For this review, use the dimensioned drawing (mm, ordinates from the lowest corner) and the shaded views. A direction names the side the tool comes from. Give positions to 0.01 mm unless a question says otherwise; leave off trailing zeros. Order: outer loops, then holes, each group sorted by start corner. A loop starts at its lowest first (then second) coordinate and runs counter-clockwise, first axis right, second up. Notation, with made-up numbers: (41, 84) - (87, 84) arc R19 ccw to (87, 99) - close; hole circle Ø10 at (79, 23). An arc over 180 degrees is marked (long way). Use a Markdown table: item, result. Add a question column.
1) We need section D-D on y = 24.5. Write out the cut boundary in (x, z), then the cut area to 3 significant figures.
2) We need section A-A on y = 39.5. Write out the cut boundary in (x, z).
3) Machinability: for the marked faces 1, 2, 3, 4 and 5, which of the approach directions +Z, -Z, +X, -X, +Y, -Y give a long, thin tool a straight path to every point of the face, cutting with its end or side? Answer none if there is none.
4) Clearance check with flat-ended pins moving along their axes: P1, Ø20.5, axis at y = 50, z = 43, coming from the +X side; P2, Ø1, axis at x = 47.5, y = 33.5, coming from the -Z side; P3, Ø15, axis at y = 47.5, z = 35, coming from the -X side. State where each tip first meets the part, or that it passes through.
5) We need section B-B on z = 65.5. Write out the cut boundary in (x, y), then the cut area to 3 significant figures.
6) We need section C-C on x = 20. Write out the cut boundary in (y, z), then the cut area to 3 significant figures.
7) Wall thickness on L1, parallel to Y at x = 94, z = 67.5; L2, parallel to Z at x = 58, y = 24; L3, parallel to Z at x = 133, y = 18: over which ranges is each line inside the solid? List them lowest first.
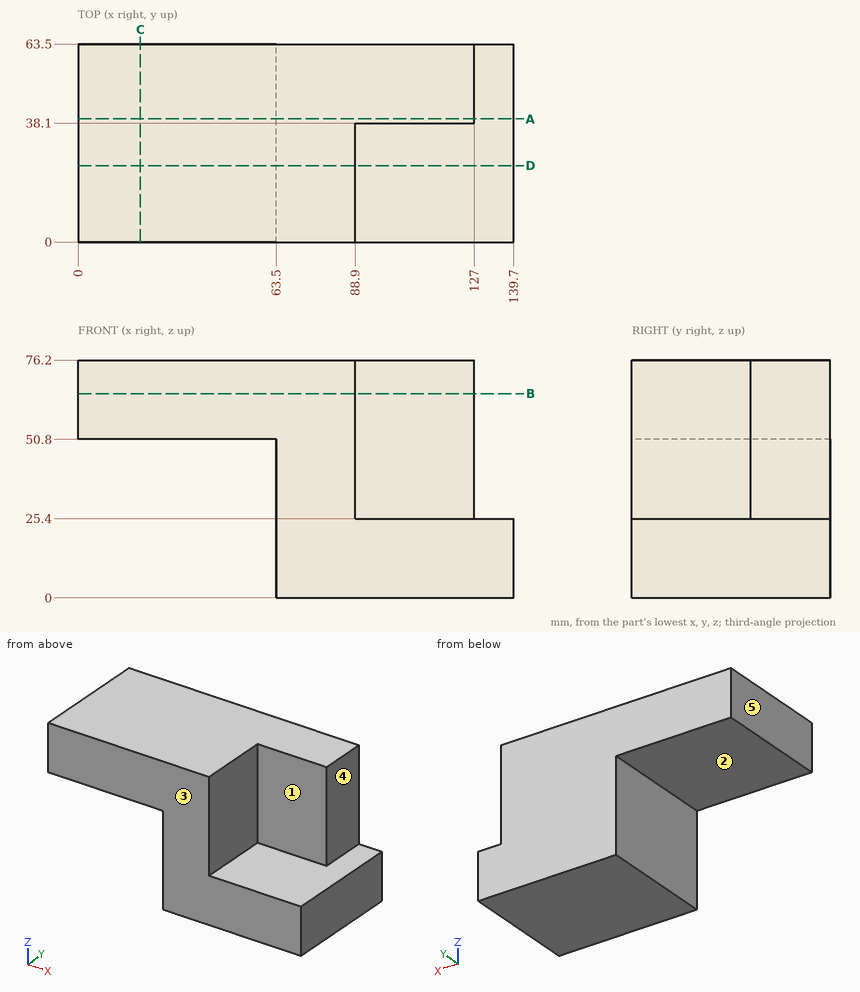
Checked values:
| question | item | result |
|---|---|---|
| 1 | outline | (0, 50.8) - (63.5, 50.8) - (63.5, 0) - (139.7, 0) - (139.7, 25.4) - (88.9, 25.4) - (88.9, 76.2) - (0, 76.2) - close |
| 1 | area | 4,840 mm² |
| 2 | outline | (0, 50.8) - (63.5, 50.8) - (63.5, 0) - (139.7, 0) - (139.7, 25.4) - (127, 25.4) - (127, 76.2) - (0, 76.2) - close |
| 3 | face 1 | +Z, +X, -Y |
| 3 | face 2 | -Z, -X, +Y, -Y |
| 3 | face 3 | +Z, -Z, +X, -X, -Y |
| 3 | face 4 | +Z, +X, +Y, -Y |
| 3 | face 5 | +Z, -Z, -X, +Y, -Y |
| 4 | P1 | x = 127 |
| 4 | P2 | z = 50.8 |
| 4 | P3 | x = 63.5 |
| 5 | outline | (0, 0) - (88.9, 0) - (88.9, 38.1) - (127, 38.1) - (127, 63.5) - (0, 63.5) - close |
| 5 | area | 6,610 mm² |
| 6 | outline | (0, 50.8) - (63.5, 50.8) - (63.5, 76.2) - (0, 76.2) - close |
| 6 | area | 1,610 mm² |
| 7 | L1 | 38.1 to 63.5 |
| 7 | L2 | 50.8 to 76.2 |
| 7 | L3 | 0 to 25.4 |
